Model file for the job. Use its own axes, mm. A direction names the side the tool comes from. Round coordinates to 2 decimals unless told otherwise and drop trailing zeros. Write each loop counter-clockwise with the first axis right and the second up, starting at its lowest first coordinate (ties: lowest second). Pieces come first, ordered by that corner, then holes. Notation, with made-up numbers: (24.5, 44.25) - (46.5, 44.25) arc R37 cw to (46.5, 83.25) - close; hole circle Ø8 at (72, 84). An arc over 180 degrees is marked (long way). One line per item, written item: value.
from build123d import *

# Parameters (mm, degrees)
F1_DEPTH = 5
F2_DEPTH = 2


with BuildPart() as f1:
    # F0 (on Top) → F1 (new body)
    with BuildSketch(Plane.XY):
        Polygon((-19.2634474565, -6.1269301263), (-18.2925394874, -3.0197121847), (-14.6755642361, 8.5557725694), (-12.6898871528, 9.0006510417), (-12.6898871528, 10.2376302083), (-20.0466579861, 10.2376302083), (-20.0466579861, 9.0006510417), (-17.1820746528, 8.5557725694), (-21.2022569444, -4.9533420139), (-26.5407986111, 8.30078125), (-28.662109375, 8.30078125), (-33.984375, -4.9913194444), (-38.8346354167, 8.5557725694), (-36.1707899306, 9.0006510417), (-36.1707899306, 10.2376302083), (-46.3758680556, 10.2376302083), (-46.3758680556, 9.0006510417), (-44.3956163194, 8.5557725694), (-36.865234375, -13.0262586806), (-34.7819010417, -13.0262586806), (-29.1666666667, 0.9982638889), (-23.5080295139, -13.0262586806), (-21.4192708333, -13.0262586806), align=None)
        Polygon((-43.2690681627, 7.6009020128), (-41.0144999623, 8.3526074886), (-35.0183658302, -8.1367557868), (-37.251050357, -8.9486413444), align=None, mode=Mode.SUBTRACT)
        Polygon((-29.3969921768, 5.0547351129), (-27.0734913647, 5.9541547671), (-21.5270686895, -8.1367557868), (-24.2253281176, -8.1367557868), align=None, mode=Mode.SUBTRACT)
        Polygon((-4.6070118818, 3.644027612), (-3.3984823364, 6.814897888), (-18.2925394874, -3.0197121847), (-19.2634474565, -6.1269301263), align=None)
        Polygon((-2.0236545139, 10.4220920139), (-3.3984823364, 6.814897888), (-4.6070118818, 3.644027612), (-10.1128472222, -10.8018663194), (-11.8055555556, -11.2630208333), (-11.8055555556, -12.5), (-4.8882378472, -12.5), (-4.8882378472, -11.2630208333), (-7.8070746528, -10.8018663194), (-5.7237413194, -4.9207899306), (3.0110677083, -4.9207899306), (5.1812065972, -10.8018663194), (2.5499131944, -11.2630208333), (2.5499131944, -12.5), (12.6736111111, -12.5), (12.6736111111, -11.2630208333), (10.9429253472, -10.8018663194), (8.5519227834, -4.4988999923), (7.5429662144, -1.8391708158), (2.8917100694, 10.4220920139), align=None)
        Polygon((-5.0238715278, -3.0544704861), (-1.2803819444, 6.9986979167), (2.3654513889, -3.0544704861), align=None, mode=Mode.SUBTRACT)
        Polygon((-0.8333516307, 7.6009020128), (2.2724873852, 8.3526074886), (10.1284366101, -10.9029943123), (6.6572050564, -10.9029943123), align=None, mode=Mode.SUBTRACT)
        Polygon((16.4388020833, 6.1594187407), (7.5429662144, -1.8391708158), (8.5519227834, -4.4988999923), (16.4388020833, 2.5924977505), align=None)
        Polygon((16.4388020833, 8.5557725694), (16.4388020833, 6.1594187407), (16.4388020833, 2.5924977505), (16.4388020833, -10.8018663194), (13.5199652778, -11.2630208333), (13.5199652778, -12.5), (21.6091579861, -12.5), (21.6091579861, -11.2630208333), (18.5601128472, -10.8018663194), (18.5601128472, 6.7111545139), (26.9476996528, -12.5), (27.880859375, -12.5), (36.4420572917, 6.7111545139), (36.4420572917, -10.8018663194), (33.3930121528, -11.2630208333), (33.3930121528, -12.5), (44.6994357639, -12.5), (44.6994357639, -11.2630208333), (41.7860243056, -10.8018663194), (41.7860243056, 8.5557725694), (44.6994357639, 9.0006510417), (44.6994357639, 10.2376302083), (35.5794270833, 10.2376302083), (28.9496527778, -4.7200520833), (22.4555121528, 10.2376302083), (13.5199652778, 10.2376302083), (13.5199652778, 9.0006510417), align=None)
        Polygon((37.6935936511, -10.9029943123), (37.6935936511, 5.9541547671), (39.3697134069, 8.3526074886), (39.3697134069, -11.9900868907), align=None, mode=Mode.SUBTRACT)
        Polygon((27.211471604, -9.1471979388), (20.3785393387, 7.6009020128), (29.0340669453, -6.3370526768), align=None, mode=Mode.SUBTRACT)
    extrude(amount=F1_DEPTH)

    # F0 (on Top) → F2 (join)
    with BuildSketch(Plane.XY):
        Polygon((-21.5270686895, -8.1367557868), (-27.0734913647, 5.9541547671), (-29.3969921768, 5.0547351129), (-24.2253281176, -8.1367557868), align=None)
        Polygon((-35.0183658302, -8.1367557868), (-41.0144999623, 8.3526074886), (-43.2690681627, 7.6009020128), (-37.251050357, -8.9486413444), align=None)
        Polygon((10.1284366101, -10.9029943123), (2.2724873852, 8.3526074886), (-0.8333516307, 7.6009020128), (6.6572050564, -10.9029943123), align=None)
        Polygon((2.3654513889, -3.0544704861), (-1.2803819444, 6.9986979167), (-5.0238715278, -3.0544704861), align=None)
        Polygon((29.0340669453, -6.3370526768), (20.3785393387, 7.6009020128), (27.211471604, -9.1471979388), align=None)
        Polygon((39.3697134069, 8.3526074886), (37.6935936511, 5.9541547671), (37.6935936511, -10.9029943123), (39.3697134069, -11.9900868907), align=None)
    extrude(amount=F2_DEPTH)


solid = f1.part
1. Tool access for faces 1 (the face through (2, 0, 5)), 2 (the face through (-16, 10.238, 2)), 3 (the face through (39, -2, 2)), 4 (the face through (-37.521, 8.775, 2.465)): list every direction of +Z, -Z, +X, -X, +Y, -Y with a clear straight run to the whole face (end or side of a thin tool).
Report:
face 1: +Z, +X, -X, +Y, -Y
face 2: +Z, -Z, -X, +Y
face 3: +Z
face 4: +Z, -Z
2. Mould opens along X. For faces 5 (the face through (-19.164, 1.896, 2.465)), 6 (the face through (39, -12.5, 2)), 7 (the face through (-40.683, -2.084, 2.465)) say: released by +X, released by -X, zero draft, split by the parting line, or undercut.
Report:
face 5: undercut
face 6: zero draft
face 7: released by -X
3. Band-saw the part on A-A on x = -13.5. Write the cut outline in (y, z).
Report:
outline: (-2.28, 0) - (0.14, 0) - (0.14, 5) - (-2.28, 5) - close; (8.82, 0) - (10.24, 0) - (10.24, 5) - (8.82, 5) - close
4. Wall check: probe 1 along X at (y, z) = (8.5, 2.3); probe 2 along Y at (x, z) = (39.5, 3.55); probe 3 along Y at (x, z) = (33.5, 3.6). Give the ranges that are in metal, low to high. Write a range as [from, to].
Report:
probe 1: [-44.38, -38.81], [-17.2, -14.69], [-2.76, 3.62], [16.44, 23.21], [34.81, 41.79]
probe 2: [-12.5, 10.24]
probe 3: [-12.5, -11.25], [0.11, 5.55]
5. Drop flat-ended pins along their axis: pin 1 (1.5 mm diameter, centred on x = 18, z = 1.5, fed in from +Y); pin 2 (0.9 mm diameter, centred on y = -2, z = 3, fed in from -X); pin 3 (0.6 mm diameter, centred on x = -27, z = 3, fed in from +Y). Give the stop position or say it passes through.
Report:
pin 1: y = 10.24
pin 2: x = -40.87
pin 3: y = 8.3
6. Band-saw the part on B-B on x = 25. Write the cut outline in (y, z), plus the area to 3 significant figures.
Report:
outline: (-8.04, 0) - (4.38, 0) - (4.38, 5) - (0.16, 5) - (0.16, 2) - (-3.73, 2) - (-3.73, 5) - (-8.04, 5) - close
area: 50.4 mm²
